The listing builds one solid part. Answer for the finished solid, in the listing's coordinates (mm). A direction names the side the tool comes from. Give positions to 0.01 mm unless a question says otherwise; leave off trailing zeros. Loops run counter-clockwise (first coordinate to the right, second up) from the corner with the lowest first, then second, coordinate; pieces in that order, holes last. Notation, with made-up numbers: M 10,-30.5 L 32,-30.5 A12 ccw 32,-17.5 Z; hole C 70,16 d5. An arc over 180 degrees is marked long. Use one line per item in the form item = value. Start each with the question number.
1. Straight lines are drawn through the part: line 1 (Y direction, x = -43.5, z = -14); line 2 (Y direction, x = 1, z = 1); line 3 (Y direction, x = 3, z = 37.5). For each, find the intervals that lie inside material, in ascending order. Write a range as from..to.
2. For faces 4 (the face through (-1.487, -74.736, -6.695)), 5 (the face through (-1.487, 74.694, -6.695)), determine the directions among +Z, -Z, +X, -X, +Y, -Y from which every point of the face is accessible in a straight line to the end or side of a thin tool.
3. The part is cut by section A-A (y = -5.5). Write down the section's boundary in (x, z), and give its area (3 significant figures).
4. Each of these flat-tipped pins is pushed along its axis until it touches: pin 1 Ø8 at (x, y) = (-7, -17.5) entering from +Z; pin 2 Ø6 at (y, z) = (-50, 2) entering from -X; pin 3 Ø24.5 at (x, z) = (-17, 17) entering from +Y. Where does it stop, or does it pass through?
5. The part is cut by section B-B (y = -53). Write down the section's boundary in (x, z).
6. The mould has two halves that part along Y. Classify faces 1 (the face through (0, -76.2, -1)), 2 (the face through (0, 76.2, -1)), 3 (the face through (-1.487, -0.48, -6.695)): released by +Y, released by -Y, zero draft, split by the parting line, or undercut.
from build123d import *

# Parameters (mm, degrees)
F0_R          = 6.858
F1_DEPTH      = 76.2
F1_DEPTH_BACK = 76.2


with BuildPart() as f1:
    # F0 (on Front) → F1 (new body, two sides)
    with BuildSketch(Plane.XZ) as f1_sk:
        Circle(F0_R)
    extrude(amount=F1_DEPTH)
    extrude(f1_sk.sketch, amount=-F1_DEPTH_BACK)

    # F2 (on Right) → F3 (revolve)
    with BuildSketch(Plane.YZ):
        with BuildLine():
            Line((-57.759602, 0), (-34.290001, 0))
            Line((-34.290001, 0), (-34.290001, 40.8432))
            ThreePointArc((-34.290001, 40.8432), (-46.024801, 48.215831), (-57.759602, 40.8432))
            Line((-57.759602, 40.8432), (-57.759602, 0))
        make_face()
    revolve(axis=Axis((0, -46.024801, 0), (0, 1, 0)))

    # F2 (on Right) → F4 (revolve)
    with BuildSketch(Plane.YZ):
        with BuildLine():
            Line((57.759602, 0), (34.290001, 0))
            Line((34.290001, 0), (34.290001, -40.8432))
            ThreePointArc((34.290001, -40.8432), (46.024801, -48.215831), (57.759602, -40.8432))
            Line((57.759602, -40.8432), (57.759602, 0))
        make_face()
    revolve(axis=Axis((0, 46.024801, 0), (0, -1, 0)))

    # F2 (on Right) → F5 (revolve)
    with BuildSketch(Plane.YZ):
        Polygon((76.352403, 0), (57.759602, 0), (57.759602, -40.8432), align=None)
    revolve(axis=Axis((0, 67.056002, 0), (0, -1, 0)))

    # F2 (on Right) → F6 (revolve)
    with BuildSketch(Plane.YZ):
        Polygon((-76.352403, 0), (-57.759602, 0), (-57.759602, 40.8432), align=None)
    revolve(axis=Axis((0, -67.056002, 0), (0, -1, 0)))


solid = f1.part
Derived:
q1.line_1 = -53.72..-38.33, 38.33..53.72
q1.line_2 = -76.2..76.2
q1.line_3 = -59.23..-34.29, 34.29..59.23
q2.face_4 = -Y
q2.face_5 = +Y
q3.outline = C 0,0 d13.72
q3.area = 148 mm2
q4.pin_1 = 6.17
q4.pin_2 = -48.16
q4.pin_3 = 70.98
q5.outline = C 0,0 d92.38
q6.face_1 = released by -Y
q6.face_2 = released by +Y
q6.face_3 = undercut
